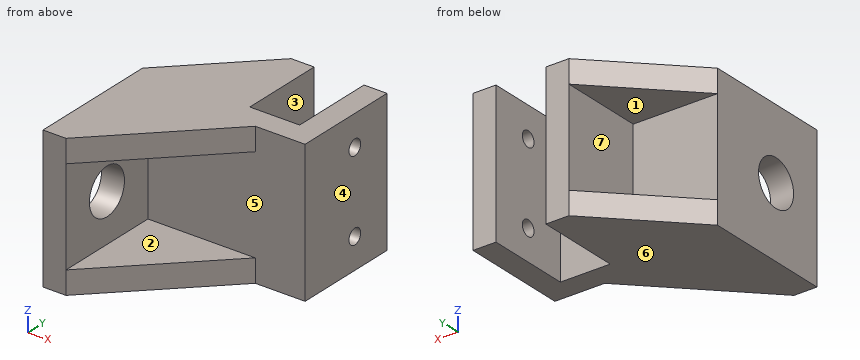
from build123d import *

# Parameters (mm, degrees)
PAD_DEPTH       = 37
PAD001_DEPTH    = 6
PAD002_DEPTH    = 6
SKETCH003_R     = 6
POCKET_DEPTH    = 47.001
SKETCH004_R     = 2
POCKET001_DEPTH = 6


with BuildPart() as part:
    # Sketch → Pad (new body)
    with BuildSketch(Plane.XY):
        Polygon((0, 0), (-22, 0), (-22, -34), (-16, -34), (-16, -6), (25, -6), (25, 22), (19, 22), (19, 0), (6, 0), (6, 22), (0, 22), align=None)
    extrude(amount=PAD_DEPTH)

    # Sketch001 (on Face14 of Pad) → Pad001 (join)
    with BuildSketch(Plane.XY.offset(37)):
        Polygon((-16, -6), (-16, -34), (12, -6), (0, -6), (0, 0), (0, 22), (-22, 0), (-16, 0), align=None)
    extrude(amount=-PAD001_DEPTH)

    # Sketch002 (on Face2 of Pad001) → Pad002 (join)
    with BuildSketch(Plane(origin=(0, 0, 0), x_dir=(1, 0, 0), z_dir=(0, 0, -1))):
        Polygon((-16, 34), (-16, 0), (-22, 0), (0, -22), (0, 6), (12, 6), align=None)
    extrude(amount=-PAD002_DEPTH)

    # Sketch003 (on Face15 of Pad002) → Pocket (cut, through all)
    with BuildSketch(Plane(origin=(-22, 0, 0), x_dir=(0, -1, 0), z_dir=(-1, 0, 0))):
        with Locations((20, 18.5)):
            Circle(SKETCH003_R)
    extrude(amount=-POCKET_DEPTH, mode=Mode.SUBTRACT)

    # Sketch004 (on Face11 of Pocket) → Pocket001 (cut)
    with BuildSketch(Plane.YZ.offset(25)):
        with Locations((11, 29)):
            Circle(SKETCH004_R)
        with Locations((11, 8)):
            Circle(SKETCH004_R)
    extrude(amount=-POCKET001_DEPTH, mode=Mode.SUBTRACT)


solid = part.part
Geometry check sheet. Reference: the model listing, model coordinates, mm. Face numbers are marked on the shaded views. A direction names the side the tool comes from. Give positions to 0.01 mm unless a question says otherwise; leave off trailing zeros. Write each loop counter-clockwise with the first axis right and the second up, starting at its lowest first coordinate (ties: lowest second). Pieces come first, ordered by that corner, then holes. Notation, with made-up numbers: M 42.25,70 L 82.25,70 A23 cw 82.25,93 Z; hole C 78,83.25 d3. An arc over 180 degrees is marked long. Answer as CSV lines item,"result". Start each with the question number.
Q1. Section check B-B, the plane y = 11. Record the cut outline in (x, z), then the cut area to 3 significant figures.
Q2. Go/stop test with flat-tipped pins: pin 1 (14 mm diameter, centred on y = -20, z = 18.5, fed in from +X); pin 2 (3 mm diameter, centred on y = 11, z = 8, fed in from -X); pin 3 (3 mm diameter, centred on y = 11, z = 29, fed in from +X). Record where each tip stops, or that it passes through.
Q3. Section check C-C, the plane x = 10.5. Record the cut outline in (y, z), then the cut area to 3 significant figures.
Q4. Section check A-A, the plane z = 8. Record the cut outline in (x, y), then the cut area to 3 significant figures.
Q5. Section check D-D, the plane y = -23. Record the cut outline in (x, z), then the cut area to 3 significant figures.
Q6. Release check for a two-part mould opening along Z. For the marked faces 4, 5, 6 and 7 record: pulls with the +Z half, pulls with the -Z half, needs draft (parallel to the pull), parting line crosses it, or undercut.
Q7. Tool access check on the marked faces 1, 2 and 3. Record the directions out of +Z, -Z, +X, -X, +Y, -Y that give a thin tool (end or side, any length) a straight path to the whole face; none if there is none.
Q8. Material ranges on L1, parallel to Z at x = 21.2, y = 11; L2, parallel to X at y = 6, z = 3; L3, parallel to Z at x = -20, y = -20, recorded low to high.
Geometry says:
1,outline,"M -11,0 L 6,0 L 6,37 L -11,37 L -11,31 L 0,31 L 0,6 L -11,6 Z; M 19,0 L 25,0 L 25,6 L 19,6 Z; M 19,10 L 25,10 L 25,27 L 19,27 Z; M 19,31 L 25,31 L 25,37 L 19,37 Z"
1,area,"528 mm^2"
2,pin 1,"x = -16"
2,pin 2,"x = 0"
2,pin 3,"x = 6"
3,outline,"M -7.5,0 L 0,0 L 0,37 L -7.5,37 L -7.5,31 L -6,31 L -6,6 L -7.5,6 Z"
3,area,"240 mm^2"
4,outline,"M -22,-34 L -16,-34 L -16,-6 L 25,-6 L 25,9 L 19,9 L 19,0 L 6,0 L 6,22 L 0,22 L 0,0 L -22,0 Z; M 19,13 L 25,13 L 25,22 L 19,22 Z"
4,area,"690 mm^2"
5,outline,"M -22,0 L -5,0 L -5,6 L -16,6 L -16,13.3 L -22,13.3 Z; M -22,23.7 L -16,23.7 L -16,31 L -5,31 L -5,37 L -22,37 Z"
5,area,"292 mm^2"
6,face 4,"needs draft"
6,face 5,"undercut"
6,face 6,"pulls with the -Z half"
6,face 7,"undercut"
7,face 1,"-X, +Y"
7,face 2,"+X, -Y"
7,face 3,"+Z, -Z, +Y"
8,L1,"0 to 6, 10 to 27, 31 to 37"
8,L2,"-16 to 6, 19 to 25"
8,L3,"0 to 12.5, 24.5 to 37"
